For this review, take the finished solid that the model builds, in its own axes (mm). Face numbers are marked on the shaded views. A direction names the side the tool comes from. Coordinates: 2 decimals unless noted, no trailing zeros. Order: outer loops, then holes, each group sorted by start corner. A loop starts at its lowest first (then second) coordinate and runs counter-clockwise, first axis right, second up. Notation, with made-up numbers: (46, 66) -> (58, 66) arc R11 ccw to (58, 71) -> close; hole circle Ø1 at (10.5, -36). An arc over 180 degrees is marked (long way). Return JSON: item names as keys, results as strings. Group by question number.
Item 1: Draft analysis for pull direction X (two halves, no side actions). For the marked faces 1, 2 and 3, state which applies: +X half, -X half, draft (parallel to the pull), parting line (faces both ways), or undercut.
Item 2: Machinability: for the marked faces 4, 5 and 6, which of the approach directions +Z, -Z, +X, -X, +Y, -Y give a long, thin tool a straight path to every point of the face, cutting with its end or side? Answer none if there is none.
Item 3: Take a section at C-C (x = 11). Write out the cut boundary in (y, z) (3 decimals), then the cut area to 3 significant figures.
Item 4: For line 1 along Z through (x, y) = (102, 2); line 2 along X through (y, z) = (0.95, -30.5); line 3 along X through (y, z) = (-6.75, -22.5), list the stretches that pass through material, from the lowest coordinate up.
Item 5: Insertion check: pin 1 (4 mm diameter, centred on x = 102, z = -14.5, fed in from -Y); pin 2 (3.5 mm diameter, centred on y = -5, z = -10.5, fed in from -X); pin 3 (4 mm diameter, centred on y = -7, z = -26.5, fed in from -X). Each pin has a flat end and moves straight along its axis. Give the tip position at first contact, or say it passes through.
Item 6: Take a section at B-B (z = -22.5). Write out the cut boundary in (x, y), then the cut area to 3 significant figures.
Item 7: Take a section at A-A (x = 48). Write out the cut boundary in (y, z), then the cut area to 3 significant figures.
```python
from build123d import *

# Parameters (mm, degrees)
SKETCH1_W                      = 113
SKETCH1_H                      = 45
BOSS_EXTRUDE1_DEPTH            = 4
M2_5_CLEARANCE_HOLE2_D         = 3.1
SKETCH5_W                      = 113
SKETCH5_H                      = 8.175
BOSS_EXTRUDE2_DEPTH            = 14
BOSS_EXTRUDE3_REACH            = 124.955
SKETCH7_W                      = 44
SKETCH7_H                      = 28.65
M2_5_CLEARANCE_HOLE1_D         = 3.1
SKETCH11_W                     = 34
SKETCH11_H                     = 35
CUT_EXTRUDE1_DEPTH             = 14
F_10_0MM_DOWEL_HOLE1_D         = 10
FILLET1_R                      = 4
CUT_EXTRUDE2_DEPTH             = 123.955276422
CUT_EXTRUDE2_DEPTH_BACK        = 14
SKETCH15_R                     = 1.6
FILLET2_R                      = 3.2
CHAMFER1_SIZE                  = 3
SKETCH20_W                     = 3
SKETCH20_H                     = 1.630303993
CUT_EXTRUDE4_DEPTH             = 123.433655504
M4_CLEARANCE_HOLE2_D           = 4.8
BOSS_EXTRUDE5_DEPTH            = 2
BOSS_EXTRUDE5_DEPTH_BACK       = 3
SKETCH29_W                     = 45
SKETCH29_H                     = 18
BOSS_EXTRUDE6_DEPTH            = 5
CHAMFER2_SIZE                  = 1.75
F_4_4_4_4_DIAMETER_HOLE1_D     = 4.4
F_4_4_4_4_DIAMETER_HOLE1_DEPTH = 5
FILLET3_R                      = 2


with BuildPart() as part:
    # Sketch1 → Boss-Extrude1 (new body)
    with BuildSketch(Plane(origin=(0, 0, 0), x_dir=(1, 0, 0), z_dir=(0, 1, 0))):
        with Locations((56.5, 22.5)):
            Rectangle(SKETCH1_W, SKETCH1_H)
    extrude(amount=BOSS_EXTRUDE1_DEPTH)

    # M2.5 Clearance Hole2 (through all)
    with Locations(Plane(origin=(0, 4, 0), x_dir=(1, 0, 0), z_dir=(0, 1, 0))):
        with Locations((11, 30.5), (23, 30.5), (23, 14.5), (11, 14.5), (102, 14.5), (90, 14.5), (90, 30.5), (102, 30.5)):
            Hole(M2_5_CLEARANCE_HOLE2_D / 2)

    # Sketch5 → Boss-Extrude2 (add)
    with BuildSketch(Plane.XZ):
        with Locations((56.5, -4.0875)):
            Rectangle(SKETCH5_W, SKETCH5_H)
        with Locations((56.5, -40.9125)):
            Rectangle(SKETCH5_W, SKETCH5_H)
    extrude(amount=BOSS_EXTRUDE2_DEPTH)

    # Sketch7 → Boss-Extrude3 (add, up to next)
    with BuildSketch(Plane.XZ.offset(14), mode=Mode.PRIVATE) as boss_extrude3_sk1:
        with Locations((56.5, -22.5)):
            Rectangle(SKETCH7_W, SKETCH7_H)
    boss_extrude3_tool1 = extrude(boss_extrude3_sk1.sketch, amount=-BOSS_EXTRUDE3_REACH, mode=Mode.PRIVATE) - part.part
    add(boss_extrude3_tool1.solids().sort_by_distance((56.5, -14, -22.5))[0])

    # M2.5 Clearance Hole1 (through all)
    with Locations(Plane(origin=(0, 0, -45), x_dir=(-1, 0, 0), z_dir=(0, 0, -1))):
        with Locations((-11, -7.25), (-23, -7.25), (-102, -7.25), (-90, -7.25)):
            Hole(M2_5_CLEARANCE_HOLE1_D / 2)

    # Sketch11 → Cut-Extrude1 (cut)
    with BuildSketch(Plane.XZ.offset(14)):
        with Locations((56.5, -22.5)):
            Rectangle(SKETCH11_W, SKETCH11_H)
    extrude(amount=-CUT_EXTRUDE1_DEPTH, mode=Mode.SUBTRACT)

    # Ø10.0mm Dowel Hole1 (through all)
    with Locations(Plane(origin=(0, 4, 0), x_dir=(1, 0, 0), z_dir=(0, 1, 0))):
        with Locations((56.5, 22.5)):
            Hole(F_10_0MM_DOWEL_HOLE1_D / 2)

    # Fillet1
    fillet1_edges = [part.edges().sort_by_distance(p)[0] for p in [
        (73.5, -7, -40),
        (39.5, -7, -40),
        (39.5, -7, -5),
        (73.5, -7, -5),
    ]]
    fillet(fillet1_edges, radius=FILLET1_R)

    # Sketch15 → Cut-Extrude2 (cut, two sides: drawn at the far end of the back side and taken through both)
    with BuildSketch(Plane.XZ.offset(14).offset(-CUT_EXTRUDE2_DEPTH_BACK)):
        with Locations((34.5, -9.775)):
            Circle(SKETCH15_R)
        with Locations((34.5, -35.225)):
            Circle(SKETCH15_R)
        with Locations((78.5, -9.775)):
            Circle(SKETCH15_R)
        with Locations((78.5, -35.225)):
            Circle(SKETCH15_R)
    extrude(amount=CUT_EXTRUDE2_DEPTH + CUT_EXTRUDE2_DEPTH_BACK, mode=Mode.SUBTRACT)

    # Fillet2
    fillet2_edges = [part.edges().sort_by_distance(p)[0] for p in [
        (78.5, -7, -33.625),
        (78.5, -7, -11.375),
        (34.5, -7, -33.625),
        (34.5, -7, -11.375),
    ]]
    fillet(fillet2_edges, radius=FILLET2_R)

    # Chamfer1
    chamfer1_edges = [part.edges().sort_by_distance(p)[0] for p in [
        (113, -14, -40.9125),
        (113, -14, -4.0875),
        (0, -14, -40.9125),
        (0, -14, -4.0875),
    ]]
    chamfer(chamfer1_edges, length=CHAMFER1_SIZE)

    # Sketch20 → Cut-Extrude4 (cut, through all)
    with BuildSketch(Plane.XZ):
        with Locations((56.5, -16.915151997)):
            Rectangle(SKETCH20_W, SKETCH20_H)
    extrude(amount=-CUT_EXTRUDE4_DEPTH, mode=Mode.SUBTRACT)

    # M4 Clearance Hole2 (through all)
    with Locations(Plane(origin=(0, 0, 0), x_dir=(-1, 0, 0), z_dir=(0, -1, 0))):
        with Locations((-48, 22.5), (-65, 22.5)):
            Hole(M4_CLEARANCE_HOLE2_D / 2)

    # Sketch28 → Boss-Extrude5 (add, two sides: drawn at the far end of the back side and taken through both)
    with BuildSketch(Plane(origin=(113, 0, 0), x_dir=(0, 0, -1), z_dir=(1, 0, 0)).offset(-BOSS_EXTRUDE5_DEPTH_BACK)):
        Polygon((45, -14), (45, -11), (45, 4), (0, 4), (0, -11), (0, -14), (8.175, -14), (8.175, -11), (8.175, 0), (36.825, 0), (36.825, -11), (36.825, -14), align=None)
    extrude(amount=BOSS_EXTRUDE5_DEPTH + BOSS_EXTRUDE5_DEPTH_BACK)

    # Sketch29 → Boss-Extrude6 (add)
    with BuildSketch(Plane(origin=(115, 0, 0), x_dir=(0, 0, -1), z_dir=(1, 0, 0))):
        with Locations((22.5, -5)):
            Rectangle(SKETCH29_W, SKETCH29_H)
    extrude(amount=BOSS_EXTRUDE6_DEPTH)

    # Chamfer2
    chamfer2_edges = [part.edges().sort_by_distance(p)[0] for p in [
        (115, -7, -8.175),
        (115, -7, -36.825),
    ]]
    chamfer(chamfer2_edges, length=CHAMFER2_SIZE)

    # Ø4.4 (4.4) Diameter Hole1
    with Locations(Plane(origin=(120, 0, 0), x_dir=(0, 0, -1), z_dir=(1, 0, 0))):
        with Locations((34.5, -5), (10.5, -5)):
            Hole(F_4_4_4_4_DIAMETER_HOLE1_D / 2, depth=F_4_4_4_4_DIAMETER_HOLE1_DEPTH)

    # Fillet3
    fillet3_edges = [part.edges().sort_by_distance(p)[0] for p in [
        (120, -5, 0),
        (120, -5, -45),
    ]]
    fillet(fillet3_edges, radius=FILLET3_R)


solid = part.part
```
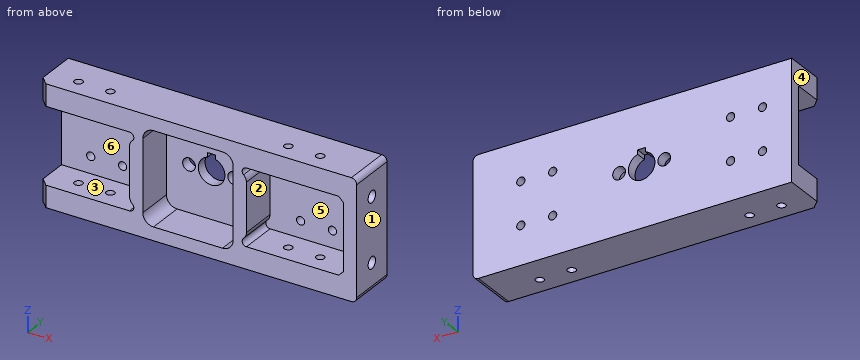
Findings below:
{
 "1": {"face 1": "+X half", "face 2": "undercut", "face 3": "draft"},
 "2": {"face 4": "+Z, -Z, -X, +Y, -Y", "face 5": "-Y", "face 6": "-X, -Y"},
 "3": {"outline": "(-14, -45) -> (-8.8, -45) -> (-8.8, -36.825) -> (-14, -36.825) -> close; (-14, -8.175) -> (-8.8, -8.175) -> (-8.8, 0) -> (-14, 0) -> close; (-5.7, -45) -> (4, -45) -> (4, -32.05) -> (0, -32.05) -> (0, -36.825) -> (-5.7, -36.825) -> close; (-5.7, -8.175) -> (0, -8.175) -> (0, -12.95) -> (4, -12.95) -> (4, 0) -> (-5.7, 0) -> close; (0, -28.95) -> (4, -28.95) -> (4, -16.05) -> (0, -16.05) -> close", "area": "333 mm2"},
 "4": {"line 1": "z = -45 to -32.05, -28.95 to -16.05, -12.95 to 0", "line 2": "x = 0 to 9.45, 12.55 to 21.45, 24.55 to 88.45, 91.55 to 100.45, 103.55 to 120", "line 3": "x = 34.5 to 39.5, 73.5 to 78.5, 115 to 120"},
 "5": {"pin 1": "stops at y = 0", "pin 2": "stops at x = 34.7", "pin 3": "stops at x = 34.5"},
 "6": {"outline": "(0, 0) -> (34.5, 0) -> (34.5, -14) -> (39.5, -14) -> (39.5, 0) -> (45.6, 0) -> (45.6, 4) -> (0, 4) -> close; (50.4, 0) -> (51.5, 0) -> (51.5, 4) -> (50.4, 4) -> close; (61.5, 0) -> (62.6, 0) -> (62.6, 4) -> (61.5, 4) -> close; (67.4, 0) -> (73.5, 0) -> (73.5, -14) -> (78.5, -14) -> (78.5, 0) -> (115, 0) -> (115, -14) -> (120, -14) -> (120, 4) -> (67.4, 4) -> close", "area": "612 mm2"},
 "7": {"outline": "(-14, -45) -> (4, -45) -> (4, -24.9) -> (0, -24.9) -> (0, -40) -> (-14, -40) -> close; (-14, -5) -> (0, -5) -> (0, -20.1) -> (4, -20.1) -> (4, 0) -> (-14, 0) -> close", "area": "301 mm2"}
}
